For this review, take the finished solid that the model builds, in its own axes (mm). A direction names the side the tool comes from. Give positions to 0.01 mm unless a question says otherwise; leave off trailing zeros. Loops run counter-clockwise (first coordinate to the right, second up) from the corner with the lowest first, then second, coordinate; pieces in that order, holes last.
```python
from build123d import *

# Parameters (mm, degrees)
SKETCH1_W             = 15.5
SKETCH1_H             = 62
BOSS_EXTRUDE1_DEPTH   = 68
FILLET1_R             = 3
CUT_EXTRUDE1_REACH    = 77.327
CUT_EXTRUDE2_DEPTH    = 48
FILLET2_R             = 5
M6_TAPPED_HOLE1_D     = 5
M6_TAPPED_HOLE1_DEPTH = 15
M6_TAPPED_HOLE1_TIP   = 1.502151548


with BuildPart() as part:
    # Sketch1 → Boss-Extrude1 (new body)
    with BuildSketch(Plane(origin=(0, 0, 0), x_dir=(1, 0, 0), z_dir=(0, 1, 0))):
        with Locations((-0.38, -0.37)):
            Rectangle(SKETCH1_W, SKETCH1_H)
    extrude(amount=-BOSS_EXTRUDE1_DEPTH)

    # Fillet1
    fillet1_edges = [part.edges().sort_by_distance(p)[0] for p in [
        (7.37, -34, 31.37),
        (-8.13, -34, 31.37),
        (-8.13, -34, -30.63),
        (7.37, -34, -30.63),
    ]]
    fillet(fillet1_edges, radius=FILLET1_R)

    # Sketch2 → Cut-Extrude1 (cut, up to next)
    with BuildSketch(Plane(origin=(0, 0, 0), x_dir=(1, 0, 0), z_dir=(0, 1, 0)), mode=Mode.PRIVATE) as cut_extrude1_sk1:
        with BuildLine():
            Line((-5.13, 10.63), (0.37, 10.63))
            ThreePointArc((0.37, 10.63), (1.784213562, 10.044213562), (2.37, 8.63))
            Line((2.37, 8.63), (2.37, -9.37))
            ThreePointArc((2.37, -9.37), (1.784213562, -10.784213562), (0.37, -11.37))
            Line((0.37, -11.37), (-5.13, -11.37))
            ThreePointArc((-5.13, -11.37), (-7.251320344, -12.248679656), (-8.13, -14.37))
            Line((-8.13, -14.37), (-8.13, 13.63))
            ThreePointArc((-8.13, 13.63), (-7.251320344, 11.508679656), (-5.13, 10.63))
        make_face()
    cut_extrude1_tool1 = extrude(cut_extrude1_sk1.sketch, amount=-CUT_EXTRUDE1_REACH, mode=Mode.PRIVATE) & part.part
    add(cut_extrude1_tool1.solids().sort_by_distance((-2.991251, 0, 0.37))[0], mode=Mode.SUBTRACT)

    # Sketch3 → Cut-Extrude2 (cut)
    with BuildSketch(Plane(origin=(0, -68, 0), x_dir=(1, 0, 0), z_dir=(0, 1, 0))):
        with BuildLine():
            Line((4.37, -16.37), (-8.13, -16.37))
            Line((-8.13, -16.37), (-8.13, -28.37))
            ThreePointArc((-8.13, -28.37), (-7.251320344, -30.491320344), (-5.13, -31.37))
            Line((-5.13, -31.37), (4.37, -31.37))
            ThreePointArc((4.37, -31.37), (6.491320344, -30.491320344), (7.37, -28.37))
            Line((7.37, -28.37), (7.37, -13.37))
            ThreePointArc((7.37, -13.37), (6.491320344, -15.491320344), (4.37, -16.37))
        make_face()
    cut_extrude2 = extrude(amount=CUT_EXTRUDE2_DEPTH, mode=Mode.SUBTRACT)

    # Mirror1: Cut-Extrude2 across plane
    add(cut_extrude2.mirror(Plane.XY), mode=Mode.SUBTRACT)

    # Fillet2
    # the kernel refuses this fillet: 5 mm, written as the material it adds along each edge
    with BuildSketch(Plane(origin=(4.37, -20, -16.37), x_dir=(0, -1, 0), z_dir=(-1, 0, 0)), Plane(origin=(4.37, -20, 16.37), x_dir=(0, 0, 1), z_dir=(-1, 0, 0))) as fillet2_piece_1:
        with BuildLine():
            CenterArc((FILLET2_R, -FILLET2_R), FILLET2_R, 90, 90)
            Line((0, -FILLET2_R), (0, 0))
            Line((0, 0), (FILLET2_R, 0))
        make_face()
    extrude(amount=12.5)
    with BuildSketch(Plane(origin=(4.37, -20, -13.37), x_dir=(-0.5176042277799098, 0, -0.855620163030514), z_dir=(0.855620163030514, 0, -0.5176042277799098))) as fillet2_piece_2_section:
        with BuildLine():
            CenterArc((-3 - FILLET2_R, -FILLET2_R), FILLET2_R, 0, 90)
            Line((-3, -FILLET2_R), (-3, 0))
            Line((-3, 0), (-3 - FILLET2_R, 0))
        make_face()
    fillet2_piece_2 = revolve(axis=Axis((4.37, -20, -13.37), (0, 1, 0)), revolution_arc=328.828315396, mode=Mode.PRIVATE)
    fillet2_piece_2 = split(fillet2_piece_2, bisect_by=Plane(origin=(6.644254363, -21.721658314, -10.63), z_dir=(0, 0, -1)), keep=Keep.TOP, mode=Mode.PRIVATE)
    fillet2_piece_2 = split(fillet2_piece_2, bisect_by=Plane(origin=(7.37, -21.721658314, -15.644254458), z_dir=(-1, 0, 0)), keep=Keep.TOP, mode=Mode.PRIVATE)
    add(fillet2_piece_2)
    with BuildSketch(Plane(origin=(4.37, -20, 13.37), x_dir=(-0.5176042277799098, 0, 0.855620163030514), z_dir=(0.855620163030514, 0, 0.5176042277799098))) as fillet2_piece_3_section:
        with BuildLine():
            CenterArc((-3 - FILLET2_R, FILLET2_R), FILLET2_R, 270, 90)
            Line((-3, FILLET2_R), (-3, 0))
            Line((-3, 0), (-3 - FILLET2_R, 0))
        make_face()
    fillet2_piece_3 = revolve(axis=Axis((4.37, -20, 13.37), (0, -1, 0)), revolution_arc=328.828315396, mode=Mode.PRIVATE)
    fillet2_piece_3 = split(fillet2_piece_3, bisect_by=Plane(origin=(6.644254403, -21.721658525, 11.37), z_dir=(0, 0, 1)), keep=Keep.TOP, mode=Mode.PRIVATE)
    fillet2_piece_3 = split(fillet2_piece_3, bisect_by=Plane(origin=(7.37, -21.721658525, 15.644254403), z_dir=(-1, 0, 0)), keep=Keep.TOP, mode=Mode.PRIVATE)
    add(fillet2_piece_3)

    # M6 Tapped Hole1
    with Locations(Plane(origin=(0, 0, 0), x_dir=(1, 0, 0), z_dir=(0, 1, 0))):
        with Locations((-0.38, 20.63), (-0.38, -21.37)):
            Hole(M6_TAPPED_HOLE1_D / 2, depth=M6_TAPPED_HOLE1_DEPTH)
            with Locations((0, 0, -(M6_TAPPED_HOLE1_DEPTH + M6_TAPPED_HOLE1_TIP / 2))):  # 118° drill point
                Cone(0, M6_TAPPED_HOLE1_D / 2, M6_TAPPED_HOLE1_TIP, mode=Mode.SUBTRACT)


solid = part.part
```
Item 1: Tool access review of faces 1 (the flat face through (0, -20, -26)), 2 (the cylindrical face through (6.51, -46.8, -15.47)), 3 (the cylindrical face through (1.8, -33.52, 10.77)), 4 (the cylindrical face through (-0.05, -7.6, 18.89)): name each direction out of +Z, -Z, +X, -X, +Y, -Y from which nothing blocks a thin tool from reaching the whole face with its end or side.
Answer:
face 1: -Z, +X, -X, -Y
face 2: -Z, +X, -Y
face 3: -X, +Y, -Y
face 4: +Y
Item 2: Take a section at D-D on y = -51. Give the boundary of the cut face in (x, z).
Answer:
outline: (-8.13, -16.37) - (4.37, -16.37) arc R3 ccw to (7.37, -13.37) - (7.37, 13.37) arc R3 ccw to (4.37, 16.37) - (-8.13, 16.37) - (-8.13, 14.37) arc R3 ccw to (-5.13, 11.37) - (0.37, 11.37) arc R2 cw to (2.37, 9.37) - (2.37, -8.63) arc R2 cw to (0.37, -10.63) - (-5.13, -10.63) arc R3 ccw to (-8.13, -13.63) - close
Item 3: Take a section at A-A on y = -18.5. Give the boundary of the cut face in (x, z).
Answer:
outline: (-8.13, -27.63) arc R3 ccw to (-5.13, -30.63) - (4.37, -30.63) arc R3 ccw to (7.37, -27.63) - (7.37, 28.37) arc R3 ccw to (4.37, 31.37) - (-5.13, 31.37) arc R3 ccw to (-8.13, 28.37) - (-8.13, 14.37) arc R3 ccw to (-5.13, 11.37) - (0.37, 11.37) arc R2 cw to (2.37, 9.37) - (2.37, -8.63) arc R2 cw to (0.37, -10.63) - (-5.13, -10.63) arc R3 ccw to (-8.13, -13.63) - close
Item 4: The part is to be moulded in two halves that separate along Z. For faces 5 (the flat face through (-8.13, -19, -19)), 6 (the flat face through (2.37, -34, 0)), 7 (the cylindrical face through (-0.05, -7.6, -23.11)), 8 (the flat face through (-2, -47, -16.37)), say which applies: released by +Z, released by -Z, zero draft, split by the parting line, or undercut.
Answer:
face 5: zero draft
face 6: undercut
face 7: undercut
face 8: released by -Z
Item 5: Clearance check with flat-ended pins moving along their axes: pin 1 Ø3 at (x, z) = (-5, 22.5) entering from -Y; pin 2 Ø1.6 at (x, y) = (-2, -46) entering from -Z; pin 3 Ø1.6 at (x, y) = (-1.5, -39) entering from +Z. State where each tip first meets the part, or that it passes through.
Answer:
pin 1: stops at y = -20.01
pin 2: stops at z = -16.37
pin 3: stops at z = 16.37
Item 6: Take a section at C-C on z = 5. Give the boundary of the cut face in (x, y).
Answer:
outline: (2.37, -68) - (7.37, -68) - (7.37, 0) - (2.37, 0) - close
Item 7: For L1, parallel to Z at x = -0.38, y = -5.5; L2, parallel to Z at x = -0.75, y = -37; L3, parallel to X at y = -53, z = 7, list the stretches that pass through material, from the lowest coordinate up.
Answer:
L1: z = -30.63 to -23.13, -18.13 to -10.63, 11.37 to 18.87, 23.87 to 31.37
L2: z = -16.37 to -10.63, 11.37 to 16.37
L3: x = 2.37 to 7.37
Item 8: Take a section at B-B on x = -6.5. Give the boundary of the cut face in (y, z).
Answer:
outline: (-68, -16.37) - (-25, -16.37) arc R5 cw to (-20, -21.37) - (-20, -30.3) - (0, -30.3) - (0, -10.96) - (-68, -10.96) - close; (-68, 11.7) - (0, 11.7) - (0, 31.04) - (-20, 31.04) - (-20, 21.37) arc R5 cw to (-25, 16.37) - (-68, 16.37) - close
